from build123d import *


with BuildPart() as part:
    # Sketch1 → Revolve1 (revolve)
    with BuildSketch(Plane.XY):
        with BuildLine():
            Line((9.585714286, -4.414285714), (15, -4.414285714))
            Line((15, -4.414285714), (15, 1.585714286))
            Line((15, 1.585714286), (14, 1.585714286))
            Line((14, 1.585714286), (14, -3.414285714))
            Line((14, -3.414285714), (11, -3.414285714))
            Line((11, -3.414285714), (11, -2.414285714))
            ThreePointArc((11, -2.414285714), (12, -1.414285714), (11, -0.414285714))
            Line((11, -0.414285714), (11, -0.314285714))
            ThreePointArc((11, -0.314285714), (10.882842712, -0.031443002), (10.6, 0.085714286))
            Line((10.6, 0.085714286), (9.024464786, 0.085714286))
            Line((9.024464786, 0.085714286), (8.024464786, -1.164285714))
            Line((8.024464786, -1.164285714), (9.585714286, -2.414285714))
            Line((9.585714286, -2.414285714), (9.585714286, -4.414285714))
        make_face()
    revolve(axis=Axis((0, 14.828571429, 0), (0, -1, 0)))


solid = part.part
Verification items for the finished model (mm, model axes). A direction names the side the tool comes from. Round coordinates to 2 decimals unless told otherwise and drop trailing zeros. Order: outer loops, then holes, each group sorted by start corner. A loop starts at its lowest first (then second) coordinate and runs counter-clockwise, first axis right, second up. Notation, with made-up numbers: (25, -22) -> (31, -22) arc R17 cw to (31, 11) -> close; hole circle Ø7 at (71, -5). An arc over 180 degrees is marked (long way). Put each result on its own line as item: value.
1) Section check A-A (z = 0). Record the cut outline in (x, y).
Final values:
outline: (-15, -4.41) -> (-9.59, -4.41) -> (-9.59, -2.41) -> (-8.02, -1.16) -> (-9.02, 0.09) -> (-10.6, 0.09) arc R0.4 ccw to (-11, -0.31) -> (-11, -0.41) arc R1 ccw to (-11, -2.41) -> (-11, -3.41) -> (-14, -3.41) -> (-14, 1.59) -> (-15, 1.59) -> close; (8.02, -1.16) -> (9.59, -2.41) -> (9.59, -4.41) -> (15, -4.41) -> (15, 1.59) -> (14, 1.59) -> (14, -3.41) -> (11, -3.41) -> (11, -2.41) arc R1 ccw to (11, -0.41) -> (11, -0.31) arc R0.4 ccw to (10.6, 0.09) -> (9.02, 0.09) -> close
2) Material ranges on line 1 (Z direction, x = 1.5, y = -2.75); line 2 (Z direction, x = 10.5, y = -1); line 3 (Z direction, x = 0.5, y = 0), recorded low to high.
Final values:
line 1: z = -14.92 to -13.92, -10.9 to -9.47, 9.47 to 10.9, 13.92 to 14.92
line 2: z = -10.71 to -9.26, -5.62 to 5.62, 9.26 to 10.71
line 3: z = -14.99 to -13.99, -10.84 to -8.94, 8.94 to 10.84, 13.99 to 14.99
3) Section check B-B (x = 0). Record the cut outline in (y, z), then the cut area to 3 significant figures.
Final values:
outline: (-4.41, -15) -> (1.59, -15) -> (1.59, -14) -> (-3.41, -14) -> (-3.41, -11) -> (-2.41, -11) arc R1 ccw to (-0.41, -11) -> (-0.31, -11) arc R0.4 ccw to (0.09, -10.6) -> (0.09, -9.02) -> (-1.16, -8.02) -> (-2.41, -9.59) -> (-4.41, -9.59) -> close; (-4.41, 9.59) -> (-2.41, 9.59) -> (-1.16, 8.02) -> (0.09, 9.02) -> (0.09, 10.6) arc R0.4 ccw to (-0.31, 11) -> (-0.41, 11) arc R1 ccw to (-2.41, 11) -> (-3.41, 11) -> (-3.41, 14) -> (1.59, 14) -> (1.59, 15) -> (-4.41, 15) -> close
area: 38.4 mm^2
4) Section check D-D (z = -13). Record the cut outline in (x, y).
Final values:
outline: (-7.48, -4.41) -> (7.48, -4.41) -> (7.48, 1.59) -> (5.2, 1.59) -> (5.2, -3.41) -> (-5.2, -3.41) -> (-5.2, 1.59) -> (-7.48, 1.59) -> close
5) Section check C-C (y = 1). Record the cut outline in (x, z), then the cut area to 3 significant figures.
Final values:
outline: circle Ø30 at (0, 0); hole circle Ø28 at (0, 0)
area: 91.1 mm^2
6) Set-up check for faces 5 (the cylindrical face through (12.932, -0.949, -5.362)), 6 (the flat face through (6.2, -3.414, -9.3)): record each of +Z, -Z, +X, -X, +Y, -Y from which the full face is reachable in a straight line by a thin tool's end or side.
Final values:
face 5: +Y
face 6: none
7) Depth check by flat-ended pin: pin 1 (10.5 mm diameter, centred on x = -2.5, z = 3, fed in from +Y); pin 2 (1 mm diameter, centred on x = 4, y = 1, fed in from +Z). Enter the tip coordinate at first touch or a pass-through.
Final values:
pin 1: stops at y = 0.09
pin 2: stops at z = 14.59
8) Mould release check, pull along Z, two halves, no side actions. Record for faces 1 (the flat face through (0, -4.414, -10)), 2 (the cylindrical face through (-2.38, -2.91, -10.74)), 3 (the cylindrical face through (-14.985, -1.372, 0.66)), 4 (the cylindrical face through (-1.248, -3.428, 9.504)): +Z half, -Z half, draft (parallel to the pull), parting line (faces both ways), or undercut.
Final values:
face 1: draft
face 2: undercut
face 3: parting line
face 4: undercut
